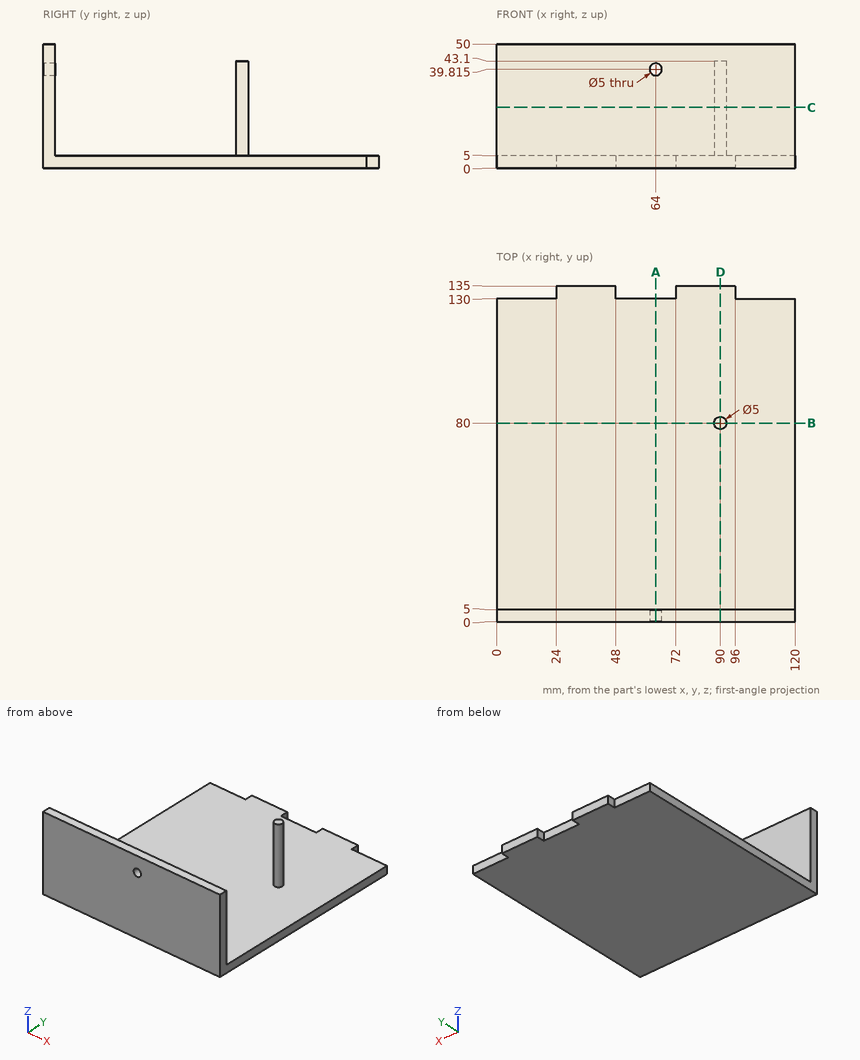
Input: dimensioned drawing with shaded views. Units: mm. Origin: part minimum x, y, z. Round coordinates to 2 decimals unless told otherwise and drop trailing zeros. Write each loop counter-clockwise with the first axis right and the second up, starting at its lowest first coordinate (ties: lowest second). Pieces come first, ordered by that corner, then holes. Notation, with made-up numbers: (-26, -38.75) - (10, -38.75) arc R10 ccw to (10, -20.75) - close; hole circle Ø1 at (-17.75, 21.5). An arc over 180 degrees is marked (long way). Write item = value, one per line.
(1) Contact query for flat-ended pins moving along their axis: pin 1 Ø4 at (x, z) = (103.5, 3.5) entering from +Y; pin 2 Ø22.5 at (x, z) = (72.5, 38) entering from +Y; pin 3 Ø2 at (x, y) = (70.5, 114) entering from +Z. Output: stop coordinate, or through.
Geometry check:
pin_1 = 130
pin_2 = 5
pin_3 = 5
(2) Section query B-B on y = 80. Output: boundary loops of the cut face in (x, z).
Geometry check:
outline = (0, 0) - (120, 0) - (120, 5) - (92.5, 5) - (92.5, 43.1) - (87.5, 43.1) - (87.5, 5) - (0, 5) - close
(3) Material intervals for probe 1 along Z at (x, y) = (64, 2) (3 decimals); probe 2 along Y at (x, z) = (17.5, 11), sorted ascending.
Geometry check:
probe_1 = 0 to 37.315, 42.315 to 50
probe_2 = 0 to 5
(4) Section query A-A on x = 64. Output: boundary loops of the cut face in (y, z) (3 decimals).
Geometry check:
outline = (0, 0) - (130, 0) - (130, 5) - (5, 5) - (5, 37.315) - (0, 37.315) - close; (0, 42.315) - (5, 42.315) - (5, 50) - (0, 50) - close
(5) Section query D-D on x = 90. Output: boundary loops of the cut face in (y, z).
Geometry check:
outline = (0, 0) - (135, 0) - (135, 5) - (82.5, 5) - (82.5, 43.1) - (77.5, 43.1) - (77.5, 5) - (5, 5) - (5, 50) - (0, 50) - close
(6) Section query C-C on z = 24.5. Output: boundary loops of the cut face in (x, y).
Geometry check:
outline = (0, 0) - (120, 0) - (120, 5) - (0, 5) - close; circle Ø5 at (90, 80)
